```python
from build123d import *

# Parameters (mm, degrees)
SKETCH_1_R      = 33.99
SKETCH_1_R_2    = 20.01
EXTRUDE_1_DEPTH = 13
CHAMFER_1_SIZE  = 1


with BuildPart() as part:
    # 草图1 → 凸台-拉伸1 (new body)
    with BuildSketch(Plane(origin=(0, 0, 0), x_dir=(1, 0, 0), z_dir=(0, 1, 0))):
        with Locations(Location((0, 0, 0), (0, 0, 90))):
            Circle(SKETCH_1_R)
        with Locations(Location((0, 0, 0), (0, 0, 90))):
            Circle(SKETCH_1_R_2, mode=Mode.SUBTRACT)
    extrude(amount=EXTRUDE_1_DEPTH)

    # 倒角1
    chamfer_1_edges = [part.edges().sort_by_distance(p)[0] for p in [
        (0, 0, 33.99),
        (0, 13, 33.99),
        (0, 0, 20.01),
        (0, 13, 20.01),
    ]]
    chamfer(chamfer_1_edges, length=CHAMFER_1_SIZE)


solid = part.part
```
Geometry: final body of the model. Coordinates: model frame, mm. Coordinates: 2 decimals unless noted, no trailing zeros. Order: outer loops, then holes, each group sorted by start corner. A loop starts at its lowest first (then second) coordinate and runs counter-clockwise, first axis right, second up.
Item 1: Section query A-A (z = 0). Output: boundary loops of the cut face in (x, y), then the cut area to 3 significant figures.
Answer:
outline: (-33.99, 1) - (-32.99, 0) - (-21.01, 0) - (-20.01, 1) - (-20.01, 12) - (-21.01, 13) - (-32.99, 13) - (-33.99, 12) - close; (20.01, 1) - (21.01, 0) - (32.99, 0) - (33.99, 1) - (33.99, 12) - (32.99, 13) - (21.01, 13) - (20.01, 12) - close
area: 359 mm2
Item 2: Draft query along X for faces 1 (the face through (22, 0, 0)), 2 (the face through (-10.21, 6.42, -32.42)), 3 (the face through (19.534, 6.423, 4.338)). Return one class per face: released by +X, released by -X, zero draft, split by the parting line, or undercut.
Answer:
face 1: zero draft
face 2: split by the parting line
face 3: undercut
Item 3: Material intervals for line 1 along X through (y, z) = (4.5, 0); line 2 along Z through (x, y) = (-15, 2); line 3 along Z through (x, y) = (-9, 3.5), sorted ascending.
Answer:
line 1: x = -33.99 to -20.01, 20.01 to 33.99
line 2: z = -30.5 to -13.24, 13.24 to 30.5
line 3: z = -32.78 to -17.87, 17.87 to 32.78
Item 4: Section query B-B (y = 4.25). Output: boundary loops of the cut face in (x, z).
Answer:
outline: circle Ø67.98 at (0, 0); hole circle Ø40.02 at (0, 0)
Item 5: Contact query for flat-ended pins moving along their axis: P1, Ø2, axis at x = 13.5, y = 5.5, coming from the -Z side; P2, Ø4, axis at x = 21.5, y = 9, coming from the +Z side; P3, Ø1.5, axis at x = 20, y = 4.5, coming from the -Z side. Output: stop coordinate, or through.
Answer:
P1: stops at z = -31.61
P2: stops at z = 27.84
P3: stops at z = -28.01
